Part model, mm, in its own coordinate system. A direction names the side the tool comes from. Round coordinates to 2 decimals unless told otherwise and drop trailing zeros. Loops run counter-clockwise (first coordinate to the right, second up) from the corner with the lowest first, then second, coordinate; pieces in that order, holes last. Notation, with made-up numbers: (62, -5.5) -> (86, -5.5) arc R20 ccw to (86, 23.5) -> close; hole circle Ø4 at (-37, 2). An arc over 180 degrees is marked (long way). Answer as a JSON object with one key per item and string values. Group by question number.
from build123d import *

# Parameters (mm, degrees)
FILLET_1_R      = 2
SKETCH_2_R      = 2
EXTRUDE_1_DEPTH = 1
FILLET_2_R      = 4


with BuildPart() as part:
    # 스케치1 → 회전1 (revolve)
    with BuildSketch(Plane.XY):
        with BuildLine():
            Line((-5.5, 15), (-7, 15))
            Line((-7, 15), (-7, 14))
            Line((-7, 14), (-14.25, 14))
            Line((-14.25, 14), (-14.25, 0))
            Line((-14.25, 0), (0, 0))
            Line((0, 0), (0, 20.5))
            ThreePointArc((0, 20.5), (-3.889087297, 18.889087297), (-5.5, 15))
        make_face()
    revolve(axis=Axis((0, 20.5, 0), (0, -1, 0)))

    # 필렛1
    fillet_1_edges = [part.edges().sort_by_distance(p)[0] for p in [
        (14.25, 14, 0),
    ]]
    fillet(fillet_1_edges, radius=FILLET_1_R)

    # 스케치2 → 보스-돌출1 (add)
    with BuildSketch(Plane(origin=(0, 0, 0), x_dir=(1, 0, 0), z_dir=(0, 1, 0))):
        Polygon((-1.166627447, 16), (-24, 2), (-24, -2), (-1.166627447, -16), (1.166627447, -16), (24, -2), (24, 2), (1.166627447, 16), align=None)
        with Locations(Location((-20, 0, 0), (0, 0, 270))):
            Circle(SKETCH_2_R, mode=Mode.SUBTRACT)
        with Locations(Location((20, 0, 0), (0, 0, 270))):
            Circle(SKETCH_2_R, mode=Mode.SUBTRACT)
    extrude(amount=-EXTRUDE_1_DEPTH)

    # 필렛2
    # the kernel refuses this fillet: 4 mm, written as the material it takes off along each edge
    with BuildSketch(Plane(origin=(24, 5.598660997, -2), x_dir=(-0.8525122061525764, 0, -0.5227073161539516), z_dir=(0, -1, 0)), Plane(origin=(24, 5.598660997, 2), x_dir=(0, 0, -1), z_dir=(0, -1, 0)), Plane(origin=(-24, 5.598660997, 2), x_dir=(0.852512206152576, 0, 0.5227073161539524), z_dir=(0, -1, 0)), Plane(origin=(-24, 5.598660997, -2), x_dir=(0, 0, 1), z_dir=(0, -1, 0))) as fillet_2_piece_1:
        with BuildLine():
            CenterArc((FILLET_2_R * 0.559866099748, -FILLET_2_R), FILLET_2_R, 90, 58.485971252)
            Line((-FILLET_2_R * 0.292646106405, -FILLET_2_R * 0.477292683846), (0, 0))
            Line((0, 0), (FILLET_2_R * 0.559866099748, 0))
        make_face()
    extrude(amount=12.197321995, mode=Mode.SUBTRACT)
    with BuildSketch(Plane(origin=(1.166627447, 2.821613344, 16), x_dir=(0.8525122061525761, 0, -0.5227073161539519), z_dir=(0, -1, 0)), Plane(origin=(1.166627447, 2.821613344, -16), x_dir=(-1, 0, 0), z_dir=(0, -1, 0)), Plane(origin=(-1.166627447, 2.821613344, -16), x_dir=(-0.8525122061525764, 0, 0.5227073161539515), z_dir=(0, -1, 0))) as fillet_2_piece_2:
        with BuildLine():
            CenterArc((FILLET_2_R * 0.28216133444, -FILLET_2_R), FILLET_2_R, 90, 31.514028748)
            Line((-FILLET_2_R * 0.240545981714, -FILLET_2_R * 0.147487793847), (0, 0))
            Line((0, 0), (FILLET_2_R * 0.28216133444, 0))
        make_face()
    extrude(amount=6.643226689, mode=Mode.SUBTRACT)
    with BuildSketch(Plane(origin=(-1.166627447, 2.821613344, 16), x_dir=(-0.8525122061525756, 0, -0.5227073161539529), z_dir=(0, -1, 0))) as fillet_2_piece_3:
        with BuildLine():
            CenterArc((FILLET_2_R * 0.28216133444, FILLET_2_R), FILLET_2_R, 238.485971252, 31.514028748)
            Line((-FILLET_2_R * 0.240545981714, FILLET_2_R * 0.147487793847), (0, 0))
            Line((0, 0), (FILLET_2_R * 0.28216133444, 0))
        make_face()
    extrude(amount=6.643226689, mode=Mode.SUBTRACT)


solid = part.part
Item 1: Two-plate mould, pull along X, no slides. Class faces 1 (the face through (-4, 15, 4)), 2 (the face through (21.983, -0.493, -0.26)), 3 (the face through (-1.109, -0.493, 15.854)): pulls with the +X half, pulls with the -X half, needs draft (parallel to the pull), parting line crosses it, or undercut.
Item 2: Band-saw the part on B-B, the plane y = 9.25. List the corners of the cut face in (x, z), plus the area to 3 significant figures.
Item 3: Which spindle directions (+Z, -Z, +X, -X, +Y, -Y) get a long thin tool onto all of the face, cutting with end or side? Do faces 4 (the face through (23.416, -0.493, -1.841)), 5 (the face through (5.3, 14, 5.3)). Say none if no direction does.
Item 4: Band-saw the part on C-C, the plane y = 12.5. List the corners of the cut face in (x, z), plus the area to 3 significant figures.
Item 5: Drop flat-ended pins along their axis: pin 1 Ø8 at (x, y) = (11, 10) entering from +Z; pin 2 Ø12 at (x, z) = (-6, 3) entering from +Y; pin 3 Ø10 at (x, y) = (12, 9.5) entering from -Z; pin 4 Ø4.5 at (x, z) = (-20, 0) entering from -Y. Give the stop position or say it passes through.
Item 6: Drill centre lines: line 1 (Y direction, x = 6, z = -2); line 2 (Y direction, x = 9.5, z = -4.5); line 3 (Z direction, x = 8.5, y = 5). Where is each one in solid material? Low to high.
Item 7: Band-saw the part on A-A, the plane x = 20. List the corners of the cut face in (y, z).
Entries:
{
 "1": {"face 1": "needs draft", "face 2": "undercut", "face 3": "pulls with the -X half"},
 "2": {"outline": "circle Ø28.5 at (0, 0)", "area": "638 mm²"},
 "3": {"face 4": "-Z, +X, +Y, -Y", "face 5": "+Y"},
 "4": {"outline": "circle Ø28.37 at (0, 0)", "area": "632 mm²"},
 "5": {"pin 1": "z = 12.41", "pin 2": "y = 20.45", "pin 3": "z = -12.41", "pin 4": "y = -1"},
 "6": {"line 1": "-1 to 15", "line 2": "-1 to 14", "line 3": "-11.44 to 11.44"},
 "7": {"outline": "(-1, -4.45) -> (0, -4.45) -> (0, -2) -> (-1, -2) -> close; (-1, 2) -> (0, 2) -> (0, 4.45) -> (-1, 4.45) -> close"}
}
